Input: part model. Units: mm. Frame: model coordinates. A direction names the side the tool comes from. Coordinates: 2 decimals unless noted, no trailing zeros. Write each loop counter-clockwise with the first axis right and the second up, starting at its lowest first coordinate (ties: lowest second). Pieces come first, ordered by that corner, then holes. Notation, with made-up numbers: (24, 29) - (33, 29) arc R10 cw to (33, 47) - close; hole circle Ø5 at (5, 87). An arc over 180 degrees is marked (long way). Put each result on its own line as item: value. Start each with the question number.
1. Access query for faces 1 (the flat face through (58, -12.5, 0)), 2 (the flat face through (-1.47, -45, 0)), 3 (the flat face through (1.47, 45, 0)), 4 (the flat face through (-3.25, 42, 0)). Directions: +Z, -Z, +X, -X, +Y, -Y. A direction counts if a zero-diameter tool reaches every point of the face in a straight line with its end or side. Return the directions, or none.
2. Cut plane C-C, the plane z = 0.9. Count the separate pieces of the cut face and the enclosed holes in it, and give its area (3 significant figures).
3. Pull-direction query (X, two-part tool) for faces 5 (the flat face through (5.475, 27, 0)), 6 (the flat face through (56.825, 31, 0)), 7 (the flat face through (-34, 50, 0)), 8 (the flat face through (-1.47, 45, 0)); classes: released by +X, released by -X, zero draft, split by the parting line, or undercut.
4. Cut plane B-B, the plane x = 11. Return loops of the section in (y, z) (1 decimal), and give its area (3 significant figures).
5. Cut plane D-D, the plane y = 14. Return loops of the section in (x, z) (1 decimal).
6. Pin query (flat end, axial travel): pin 1 (1.3 mm diameter, centred on y = -42.5, z = 1, fed in from -X) (3 decimals); pin 2 (1.3 mm diameter, centred on y = 42, z = -0.5, fed in from +X) (3 decimals); pin 3 (0.9 mm diameter, centred on x = -2.5, z = 0, fed in from -Y) (3 decimals). Return the tip coordinate at first contact, or that it passes through.
7. Line query: line 1 (Y direction, x = -2, z = 0.05) (3 decimals); line 2 (Y direction, x = 7.5, z = 0.25) (3 decimals); line 3 (X direction, y = 25, z = 0.6) (3 decimals). Output: solid intervals per line, ascending.
8. Cut plane A-A, the plane y = 0. Return loops of the section in (x, z).
from build123d import *

# Parameters (mm, degrees)
SKETCH1_R           = 1.47
BOSS_EXTRUDE1_DEPTH = 1.5875
CUT_EXTRUDE1_DEPTH  = 4.175


with BuildPart() as part:
    # Sketch1 → Boss-Extrude1 (new body, symmetric)
    with BuildSketch(Plane.XY):
        Polygon((-12.5, 50), (-56.825, 50), (-56.825, 12.5), (-60, 12.5), (-60, -12.5), (-56.825, -12.5), (-56.825, -50), (-12.5, -50), (-12.5, -46.825), (-1.47, -46.825), (-1.47, -43.125), (-3.25, -43.125), (-3.25, -40.525), (-1.47, -40.525), (-1.47, -36.825), (1.47, -36.825), (1.47, -40.525), (3.25, -40.525), (3.25, -43.125), (1.47, -43.125), (1.47, -46.825), (12.5, -46.825), (12.5, -50), (56.825, -50), (56.825, -12.5), (60, -12.5), (60, 12.5), (56.825, 12.5), (56.825, 50), (12.5, 50), (12.5, 46.825), (1.47, 46.825), (1.47, 43.125), (3.25, 43.125), (3.25, 40.525), (1.47, 40.525), (1.47, 36.825), (-1.47, 36.825), (-1.47, 40.525), (-3.25, 40.525), (-3.25, 43.125), (-1.47, 43.125), (-1.47, 46.825), (-12.5, 46.825), align=None)
        with Locations((-58.4125, 0)):
            Circle(SKETCH1_R, mode=Mode.SUBTRACT)
        with Locations((58.4125, 0)):
            Circle(SKETCH1_R, mode=Mode.SUBTRACT)
    extrude(amount=BOSS_EXTRUDE1_DEPTH, both=True)

    # Sketch2 → Cut-Extrude1 (cut, through all)
    with BuildSketch(Plane(origin=(0, 0, -1.5875), x_dir=(-1, 0, 0), z_dir=(0, 0, -1))):
        Polygon((-5.975, 32.525), (-16.975, 32.525), (-17.475, 32.525), (-17.475, 32.025), (-17.475, 22.525), (-17.475, 22.025), (-16.975, 22.025), (-5.975, 22.025), (-5.475, 22.025), (-5.475, 22.525), (-5.475, 32.025), (-5.475, 32.525), align=None)
    extrude(amount=-CUT_EXTRUDE1_DEPTH, mode=Mode.SUBTRACT)


solid = part.part
Report:
1. face 1: +Z, -Z, +X, -Y
1. face 2: +Z, -Z, -Y
1. face 3: +Z, -Z, +Y
1. face 4: +Z, -Z
2. separate pieces: 1
2. enclosed holes: 3
2. area: 11,100 mm^2
3. face 5: undercut
3. face 6: released by +X
3. face 7: zero draft
3. face 8: undercut
4. outline: (-46.8, -1.6) - (22, -1.6) - (22, 1.6) - (-46.8, 1.6) - close; (32.5, -1.6) - (46.8, -1.6) - (46.8, 1.6) - (32.5, 1.6) - close
4. area: 264 mm^2
5. outline: (-56.8, -1.6) - (56.8, -1.6) - (56.8, 1.6) - (-56.8, 1.6) - close
6. pin 1: stops at x = -56.825
6. pin 2: stops at x = 56.825
6. pin 3: stops at y = -46.825
7. line 1: y = -46.825 to -43.125, -40.525 to 40.525, 43.125 to 46.825
7. line 2: y = -46.825 to 22.025, 32.525 to 46.825
7. line 3: x = -56.825 to 5.475, 17.475 to 56.825
8. outline: (-60, -1.59) - (-59.88, -1.59) - (-59.88, 1.59) - (-60, 1.59) - close; (-56.94, -1.59) - (56.94, -1.59) - (56.94, 1.59) - (-56.94, 1.59) - close; (59.88, -1.59) - (60, -1.59) - (60, 1.59) - (59.88, 1.59) - close
